Input: part model. Units: mm. Frame: model coordinates. A direction names the side the tool comes from. Give positions to 0.01 mm unless a question says otherwise; leave off trailing zeros. Loops run counter-clockwise (first coordinate to the right, second up) from the corner with the lowest first, then second, coordinate; pieces in that order, holes last. Notation, with made-up numbers: M 74.25,-16 L 94.25,-16 A9 ccw 94.25,-7 Z; hole C 56.5,6.25 d6. An arc over 180 degrees is marked long. Answer as a JSON object with one key per item and string values. Group by question number.
1) Section query A-A on z = 15.25. Return loops of the section in (x, y).
2) Section query B-B on x = 0. Return loops of the section in (y, z), plus the area to 3 significant figures.
3) Access query for faces 1 (the flat face through (0, -12.5, 2)), 2 (the cylindrical face through (0, -2, 12)). Directions: +Z, -Z, +X, -X, +Y, -Y. A direction counts if a zero-diameter tool reaches every point of the face in a straight line with its end or side. Return the directions, or none.
4) Draft query along X for faces 3 (the flat face through (18, 0, 20)), 4 (the flat face through (30, 0, 2)), 5 (the cylindrical face through (-19.6, -1.2, 12.4)). Return one class per face: +X half, -X half, draft (parallel to the pull), parting line (faces both ways), or undercut.
5) Ray query, L1, parallel to X at y = -0.5, z = 11.5; L2, parallel to Z at x = 14.5, y = -1.5. Return the intervals inside material, ascending.
6) First-contact query: P1, Ø2, axis at x = -3.5, z = 8, coming from the +Y side; P2, Ø6, axis at x = -4, z = 12, coming from the -Y side; P3, Ø1.5, axis at x = -18.5, z = 17, coming from the +Y side. Flat tips, straight axial feed; report the tip coordinate or a pass-through.
7) Section query C-C on y = 0. Return loops of the section in (x, z).
8) Section query D-D on x = 19. Return loops of the section in (y, z), plus the area to 3 significant figures.
from build123d import *

# Parameters (mm, degrees)
F0_W     = 60
F0_H     = 25
F1_DEPTH = 5
F2_R     = 2
F3_DEPTH = 15
F4_R     = 2
F5_DEPTH = 15
F6_DEPTH = 15
F7_R     = 2
F8_DEPTH = 15


with BuildPart() as f1:
    # F0 (on Top) → F1 (new body)
    with BuildSketch(Plane.XY):
        Rectangle(F0_W, F0_H)
    extrude(amount=F1_DEPTH)

    # F2 (on face) → F3 (join)
    with BuildSketch(Plane.XY.offset(5)):
        Circle(F2_R)
    extrude(amount=F3_DEPTH)

    # F4 (on face) → F5 (join)
    with BuildSketch(Plane.XY.offset(5)):
        with Locations((18, 0)):
            Circle(F4_R)
    extrude(amount=F5_DEPTH)

    # F4 (on face) → F6 (join)
    with BuildSketch(Plane.XY.offset(5)):
        with Locations((18, 0)):
            Circle(F4_R)
    extrude(amount=F6_DEPTH)

    # F7 (on face) → F8 (join)
    with BuildSketch(Plane.XY.offset(5)):
        with Locations((-18, 0)):
            Circle(F7_R)
    extrude(amount=F8_DEPTH)


solid = f1.part
Output:
{
 "1": {"outline": "C -18,0 d4; C 0,0 d4; C 18,0 d4"},
 "2": {"outline": "M -12.5,0 L 12.5,0 L 12.5,5 L 2,5 L 2,20 L -2,20 L -2,5 L -12.5,5 Z", "area": "185 mm^2"},
 "3": {"face 1": "+Z, -Z, +X, -X, -Y", "face 2": "+Z"},
 "4": {"face 3": "draft", "face 4": "+X half", "face 5": "undercut"},
 "5": {"L1": "x = -19.94 to -16.06, -1.94 to 1.94, 16.06 to 19.94", "L2": "z = 0 to 5"},
 "6": {"P1": "passes through", "P2": "stops at y = -1.73", "P3": "stops at y = 2"},
 "7": {"outline": "M -30,0 L 30,0 L 30,5 L 20,5 L 20,20 L 16,20 L 16,5 L 2,5 L 2,20 L -2,20 L -2,5 L -16,5 L -16,20 L -20,20 L -20,5 L -30,5 Z"},
 "8": {"outline": "M -12.5,0 L 12.5,0 L 12.5,5 L 1.73,5 L 1.73,20 L -1.73,20 L -1.73,5 L -12.5,5 Z", "area": "177 mm^2"}
}
